Part model, mm, in its own coordinate system. Face numbers are marked on the shaded views. A direction names the side the tool comes from. Round coordinates to 2 decimals unless told otherwise and drop trailing zeros. Loops run counter-clockwise (first coordinate to the right, second up) from the corner with the lowest first, then second, coordinate; pieces in that order, holes last.
1) Drop flat-ended pins along their axis: P1, Ø5, axis at x = 48, z = 19.5, coming from the +Y side; P2, Ø12, axis at x = -8.5, z = 43, coming from the +Y side; P3, Ø19.5, axis at x = -34.5, z = 35, coming from the +Y side; P4, Ø11, axis at y = -7, z = -49, coming from the +X side. Give the stop position or say it passes through.
2) Probe line 1 (Z direction, x = 0, y = -18); line 2 (X direction, y = -2.5, z = 39). List the from-to ranges inside material, lowest first.
3) Band-saw the part on A-A, the plane z = 0. Write the cut outline in (x, y), then the cut area to 3 significant figures.
4) 3-axis set-ups, long thin cutter, end or side, ignore diameter. For the marked faces 1, 2 and 3: which of +Z, -Z, +X, -X, +Y, -Y reach the whole face in a straight line?
5) Band-saw the part on D-D, the plane y = -47. Write the cut outline in (x, z).
6) Band-saw the part on C-C, the plane x = -59. Write the cut outline in (y, z).
7) Band-saw the part on B-B, the plane x = 0. Write the cut outline in (y, z).
from build123d import *

# Parameters (mm, degrees)
SKETCH3_W          = 12.5
SKETCH3_H          = 12.6
CUT_EXTRUDE1_DEPTH = 10
CIRPATTERN1_COUNT  = 16
CUT_SWEEP3_ANGLE   = 46.890766


# Read off the part's stored shape, not the designer's step: Cut-Sweep3
with BuildPart() as part:
    # Sketch1 → Revolve1 (revolve)
    with BuildSketch(Plane(origin=(0, 0, 0), x_dir=(0, 0, -1), z_dir=(1, 0, 0))):
        Polygon((13.767922605, 0), (67.742922605, 0), (67.742922605, -15), (16.605833346, -15), (16.605833346, -42.092408241), (7.539548782, -80.219585538), (2.539548782, -80.219585538), (13.767922605, -33), align=None)
    revolve(axis=Axis((0, 0, 0), (0, 1, 0)))

    # Sketch3 → Cut-Extrude1 (cut)
    with BuildSketch(Plane(origin=(0, 0, 0), x_dir=(1, 0, 0), z_dir=(0, 1, 0))):
        with Locations((0, 50)):
            Rectangle(SKETCH3_W, SKETCH3_H)
    cut_extrude1 = extrude(amount=-CUT_EXTRUDE1_DEPTH, mode=Mode.SUBTRACT)

    # CirPattern1: Cut-Extrude1 ×16 about axis, 2 skipped
    cirpattern1_axis = Axis((0, 0, 0), (0, -1, 0))
    add([cut_extrude1.rotate(cirpattern1_axis, i * 360 / CIRPATTERN1_COUNT) for i in range(1, CIRPATTERN1_COUNT) if i not in (8, 9)], mode=Mode.SUBTRACT)

    # Cut-Sweep3 outline → Cut-Sweep3 (revolve, cut)
    with BuildSketch(Plane(origin=(0, 0, 0), x_dir=(-0.5705578043075069, 0, 0.8212574455941308), z_dir=(-0.8212574455941308, 0, -0.5705578043075069))):
        Polygon((54.406189133, -5), (54.406189133, 0), (13.767922605, 0), (13.767922605, -12.46941978), align=None)
    revolve(axis=Axis((0, 0, 0), (0, 1, 0)), revolution_arc=CUT_SWEEP3_ANGLE, mode=Mode.SUBTRACT)


solid = part.part
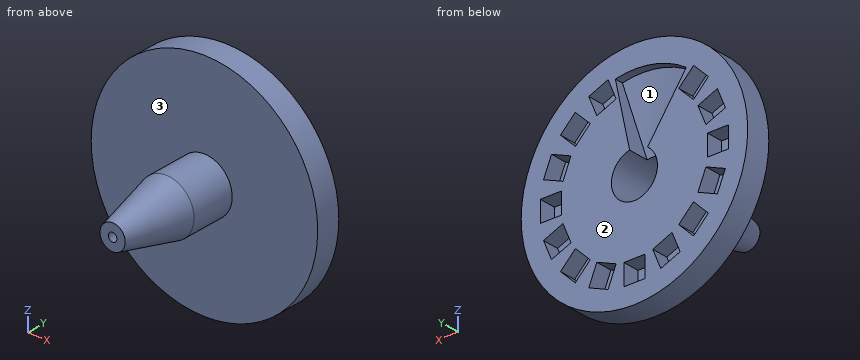
Reported:
1. P1: stops at y = -10
1. P2: stops at y = -5.84
1. P3: stops at y = 0
1. P4: stops at x = 51.93
2. line 1: z = -16.61 to -13.77, 13.77 to 16.61
2. line 2: x = -55.39 to -40.62, -30.16 to -27.09, 8.36 to 20.04, 22.92 to 30.16, 40.62 to 55.39
3. outline: (-67.74, -15) - (-16.61, -15) - (-16.61, -42.09) - (-7.54, -80.22) - (-2.54, -80.22) - (-13.77, -33) - (-13.77, 0) - (-43.7, 0) - (-43.7, -10) - (-56.3, -10) - (-56.3, 0) - (-67.74, 0) - close; (2.54, -80.22) - (7.54, -80.22) - (16.61, -42.09) - (16.61, -15) - (67.74, -15) - (67.74, 0) - (56.3, 0) - (56.3, -10) - (43.7, -10) - (43.7, 0) - (13.77, 0) - (13.77, -33) - close
3. area: 1,920 mm2
4. face 1: +Y
4. face 2: +Z, -Z, +X, -X, +Y
4. face 3: -Y
5. outline: circle Ø30.88 at (0, 0); hole circle Ø20.88 at (0, 0)
6. outline: (-15, -33.29) - (0, -33.29) - (0, 33.29) - (-15, 33.29) - close
7. outline: (-80.22, -7.54) - (-42.09, -16.61) - (-15, -16.61) - (-15, -67.74) - (0, -67.74) - (0, -56.3) - (-10, -56.3) - (-10, -43.7) - (0, -43.7) - (0, -13.77) - (-33, -13.77) - (-80.22, -2.54) - close; (-80.22, 2.54) - (-33, 13.77) - (-12.47, 13.77) - (-5, 54.41) - (0, 54.41) - (0, 67.74) - (-15, 67.74) - (-15, 16.61) - (-42.09, 16.61) - (-80.22, 7.54) - close
